Work out the finished part from the listing and answer in its coordinate system (mm). A direction names the side the tool comes from. Give positions to 0.01 mm unless a question says otherwise; leave off trailing zeros. Order: outer loops, then holes, each group sorted by start corner. A loop starts at its lowest first (then second) coordinate and runs counter-clockwise, first axis right, second up. Notation, with made-up numbers: (53.25, 15) - (59.25, 15) arc R13 cw to (59.25, 40) - close; hole circle Ø8 at (42, 52.5). An arc over 180 degrees is marked (long way). Return JSON: item names as keys, results as strings. Group by question number.
Autodesk Fusion 360 part; units mm, degrees
sketch "Sketch1" plane through (0, 0, 0) normal (0, 0, 1) x (1, 0, 0)
  line L0 (-65, 0) -> (65, 0)
  line L1 (-60, 60) -> (60, 60)
  line L2 (65, 55) -> (65, -55)
  line L3 (60, -60) -> (-60, -60)
  line L4 (-65, -55) -> (-65, 55)
  line L5 (-65, 60) -> (65, -60) construction
  line L6 (65, 60) -> (-65, -60) construction
  line L7 (-65, 0) -> (-85, 0) construction
  circle A0 centre (-75, 0) radius 3
  line L8 (0, 2.5) -> (0, 20) construction
  line L9 (65, 0) -> (85, 0) construction
  circle A1 centre (75, 0) radius 3
  line L10 (0, 60) -> (0, 80) construction
  circle A2 centre (0, 70) radius 3
  line L11 (20, 0) -> (2.5, 0)
  circle A3 centre (0, -70) radius 3
  line L12 (0, -60) -> (0, -80) construction
  circle A4 centre (-75, -50) radius 3
  circle A5 centre (-75, 50) radius 3
  circle A6 centre (75, 50) radius 3
  circle A7 centre (75, -50) radius 3
  circle A8 centre (-55, 70) radius 3
  circle A9 centre (55, 70) radius 3
  circle A10 centre (-55, -70) radius 3
  circle A11 centre (55, -70) radius 3
  line L13 (-85, 55) -> (-85, -55)
  line L14 (85, 55) -> (85, -55)
  line L15 (-60, 80) -> (60, 80)
  line L16 (-60, -80) -> (60, -80)
  circle A12 centre (49.5242, -49.6041) radius 2.5
  circle A13 centre (-0.0023, -49.6041) radius 2.5
  circle A14 centre (-49.5289, -49.6041) radius 2.5
  circle A15 centre (49.5242, 49.6459) radius 2.5
  circle A16 centre (-0.0023, 49.6459) radius 2.5
  circle A17 centre (-49.5289, 49.6459) radius 2.5
  arc A18 (-65, -55) -> (-60, -60) centre (-60, -55) ccw
  arc A19 (-60, 60) -> (-65, 55) centre (-60, 55) ccw
  arc A20 (65, 55) -> (60, 60) centre (60, 55) ccw
  arc A21 (60, -60) -> (65, -55) centre (60, -55) ccw
  line L17 (-75, 0) -> (-75, 17) construction
  line L18 (-75, 0) -> (-75, -17) construction
  circle A22 centre (-75, -17) radius 3
  circle A23 centre (-75, 17) radius 3
  circle A24 centre (75, -17) radius 3
  circle A25 centre (75, 17) radius 3
  line L19 (75, 0) -> (75, 17) construction
  line L20 (75, 0) -> (75, -17) construction
  arc A26 (-85, -55) -> (-60, -80) centre (-60, -55) ccw
  arc A27 (60, -80) -> (85, -55) centre (60, -55) ccw
  arc A28 (85, 55) -> (60, 80) centre (60, 55) ccw
  arc A29 (-60, 80) -> (-85, 55) centre (-60, 55) ccw
  point P0 (-65, 0)
  point P1 (-85, 80)
  point P2 (-85, -80)
  point P3 (85, -80)
  point P4 (85, 80)
  point P5 (-65, -80)
  point P6 (-85, -60)
  point P7 (-65, 80)
  point P8 (-85, 60)
  point P9 (65, 80)
  point P10 (85, 60)
  point P11 (85, -60)
  point P12 (65, -80)
  dimension "d30" = 65
  dimension "d31" = 130
  dimension "d32" = 120
  dimension "d33" = 20
  dimension "d34" = 6
  dimension "d35" = 20
  dimension "d36" = 6
  dimension "d39" = 0
  dimension "d40" = 50
  dimension "d43" = 55
  dimension "d44" = 0
  dimension "d45" = 5
  dimension "d46" = 5
  dimension "d47" = 5
  dimension "d48" = 20
  dimension "d49" = 20
  dimension "d50" = 20
  dimension "d51" = 20
  dimension "d52" = 20
  dimension "d53" = 20
  dimension "d54" = 20
  dimension "d55" = 20
  dimension "d56" = 5
  dimension "d60" = 17
  dimension "d63" = 0
  dimension "d64" = 17
  dimension "d65" = 25
extrude "Extrude1" add sketch "Sketch1" along normal blind 2 contours L13 L14 L15 L16 A26 A27 A28 A29
equation "d31 = 65 mm + 65 mm"
equation "d49 = d48"
equation "d51 = d50"
equation "d53 = d52"
equation "d55 = d54"
1. The part is cut by section B-B (z = 1.7). State how many separate pieces and enclosed holes the cut face has, and give its area (3 significant figures).
2. The part is cut by section A-A (y = 37). Give the vertices of the cut face in (x, z), and give its area (3 significant figures).
3. Determine the mould class of faces 3 (the cylindrical face through (52.6, -68.2, 1)), 4 (the cylindrical face through (-77.871, 72.482, 0.986)), 5 (the flat face through (6, 66, 0)), 6 (the cylindrical face through (77.871, -72.482, 0.986)) for opening direction Y: released by +Y, released by -Y, zero draft, split by the parting line, or undercut.
4. The part is cut by section C-C (y = 70). Give the vertices of the cut face in (x, z).
5. The part is cut by section D-D (x = -32). Give the vertices of the cut face in (y, z).
6. A tool of negligible diameter and unlimited length cuts with its end or side. For faces 1 (the flat face through (6, 66, 2)), 2 (the cylindrical face through (-64, 58, 1)), from which of +Z, -Z, +X, -X, +Y, -Y can it reach the whole face along a straight path? Write none if from no direction.
7. Consider probe 1 along X at (y, z) = (49.5, 1); probe 2 along Y at (x, z) = (55, 1.5); probe 3 along X at (y, z) = (68, 0.9). Determine where each line is inside the solid, lowest interval first. Write a range as from..to.
Answers:
{
 "1": {"separate pieces": "1", "enclosed holes": "17", "area": "10,600 mm^2"},
 "2": {"outline": "(-85, 0) - (-65, 0) - (-65, 2) - (-85, 2) - close; (65, 0) - (85, 0) - (85, 2) - (65, 2) - close", "area": "80.0 mm^2"},
 "3": {"face 3": "undercut", "face 4": "released by +Y", "face 5": "zero draft", "face 6": "released by -Y"},
 "4": {"outline": "(-80, 0) - (-58, 0) - (-58, 2) - (-80, 2) - close; (-52, 0) - (-3, 0) - (-3, 2) - (-52, 2) - close; (3, 0) - (52, 0) - (52, 2) - (3, 2) - close; (58, 0) - (80, 0) - (80, 2) - (58, 2) - close"},
 "5": {"outline": "(-80, 0) - (-60, 0) - (-60, 2) - (-80, 2) - close; (60, 0) - (80, 0) - (80, 2) - (60, 2) - close"},
 "6": {"face 1": "+Z, +X, -X, +Y, -Y", "face 2": "+Z, -Z"},
 "7": {"probe 1": "x = -85..-77.96, -72.04..-65, 65..72.04, 77.96..85", "probe 2": "y = -80..-73, -67..-60, 60..67, 73..80", "probe 3": "x = -81.35..-57.24, -52.76..-2.24, 2.24..52.76, 57.24..81.35"}
}
